Check sheet for the modelled part. Datum: model origin and axes. Units: mm. A direction names the side the tool comes from. Round coordinates to 2 decimals unless told otherwise and drop trailing zeros. Order: outer loops, then holes, each group sorted by start corner. A loop starts at its lowest first (then second) coordinate and runs counter-clockwise, first axis right, second up.
from build123d import *

# Parameters (mm, degrees)
SKETCH028_W     = 110
SKETCH028_H     = 32.6
PAD019_DEPTH    = 46
POCKET009_DEPTH = 19.35
SKETCH030_R     = 2.25
POCKET010_DEPTH = 5
FILLET008_R     = 3.5
SKETCH031_W     = 97
SKETCH031_H     = 2.5
POCKET011_DEPTH = 14.4
FILLET009_R     = 2
FILLET010_R     = 5
SKETCH032_W     = 25.7
SKETCH032_H     = 12.8
POCKET012_DEPTH = 11.6
SKETCH033_W     = 6.52
SKETCH033_H     = 12.8
SKETCH033_W_2   = 6.6
POCKET013_DEPTH = 22
SKETCH034_W     = 6.6
SKETCH034_H     = 15.25
SKETCH034_W_2   = 6.52
POCKET014_DEPTH = 17.55
FILLET011_R     = 1.5
SKETCH035_R     = 1.6
POCKET015_DEPTH = 5
SKETCH036_W     = 5.6
SKETCH036_H     = 2.6
POCKET016_DEPTH = 8.3
SKETCH037_W     = 5.6
SKETCH037_H     = 2.6
POCKET017_DEPTH = 8.3
PRISM_DEPTH     = 56


with BuildPart() as part:
    # Sketch028 → Pad019 (new body)
    with BuildSketch(Plane.XY):
        Rectangle(SKETCH028_W, SKETCH028_H)
    extrude(amount=PAD019_DEPTH)

    # Sketch029 (on Face6 of Pad019) → Pocket009 (cut)
    with BuildSketch(Plane.XY.offset(46)):
        Polygon((-50.7, 16.3), (-42, 16.3), (-42, 11.3), (-33, 11.3), (-33, 16.3), (33, 16.3), (33, 11.3), (42, 11.3), (42, 16.3), (50.7, 16.3), (50.7, -13.8), (-50.7, -13.8), align=None)
    extrude(amount=-POCKET009_DEPTH, mode=Mode.SUBTRACT)

    # Sketch030 (on Face1 of Pocket009) → Pocket010 (cut)
    with BuildSketch(Plane(origin=(0, 16.3, 0), x_dir=(-1, 0, 0), z_dir=(0, 1, 0))):
        with Locations((-37.5, 41.5)):
            Circle(SKETCH030_R)
        with Locations((37.5, 41.5)):
            Circle(SKETCH030_R)
    extrude(amount=-POCKET010_DEPTH, mode=Mode.SUBTRACT)

    # Fillet008
    fillet008_edges = [part.edges().sort_by_distance(p)[0] for p in [
        (33, 13.8, 46),
        (-33, 13.8, 46),
        (-42, 13.8, 46),
        (42, 13.8, 46),
    ]]
    fillet(fillet008_edges, radius=FILLET008_R)

    # Sketch031 (on Face8 of Fillet008) → Pocket011 (cut)
    with BuildSketch(Plane.XY.offset(46)):
        with Locations((0, -15.05)):
            Rectangle(SKETCH031_W, SKETCH031_H)
    extrude(amount=-POCKET011_DEPTH, mode=Mode.SUBTRACT)

    # Fillet009
    fillet009_edges = [part.edges().sort_by_distance(p)[0] for p in [
        (48.5, -15.05, 31.6),
        (-48.5, -15.05, 31.6),
    ]]
    fillet(fillet009_edges, radius=FILLET009_R)

    # Fillet010
    fillet010_edges = [part.edges().sort_by_distance(p)[0] for p in [
        (42, 13.8, 26.65),
        (-33, 13.8, 26.65),
        (33, 13.8, 26.65),
        (-42, 13.8, 26.65),
    ]]
    fillet(fillet010_edges, radius=FILLET010_R)

    # Sketch032 (on Face1 of Fillet010) → Pocket012 (cut)
    with BuildSketch(Plane.XY.offset(26.65)):
        with Locations((13.55, -5)):
            Rectangle(SKETCH032_W, SKETCH032_H)
    extrude(amount=-POCKET012_DEPTH, mode=Mode.SUBTRACT)

    # Sketch033 (on Face38 of Pocket012) → Pocket013 (cut)
    with BuildSketch(Plane.XY.offset(15.05)):
        with Locations((5.51, -5)):
            Rectangle(SKETCH033_W, SKETCH033_H)
        with Locations((21.58, -5)):
            Rectangle(SKETCH033_W_2, SKETCH033_H)
    extrude(amount=-POCKET013_DEPTH, mode=Mode.SUBTRACT)

    # Sketch034 (on Face2 of Pocket013) → Pocket014 (cut)
    with BuildSketch(Plane(origin=(0, 16.3, 0), x_dir=(-1, 0, 0), z_dir=(0, 1, 0))):
        with Locations((-21.58, 7.625)):
            Rectangle(SKETCH034_W, SKETCH034_H)
        with Locations((-5.51, 7.625)):
            Rectangle(SKETCH034_W_2, SKETCH034_H)
    extrude(amount=-POCKET014_DEPTH, mode=Mode.SUBTRACT)

    # Fillet011
    fillet011_edges = [part.edges().sort_by_distance(p)[0] for p in [
        (0.7, 1.4, 20.85),
        (26.4, -11.4, 20.85),
        (0.7, -11.4, 20.85),
        (26.4, 1.4, 20.85),
        (24.88, 16.3, 7.625),
        (18.28, 16.3, 7.625),
        (8.77, 16.3, 7.625),
        (2.25, 16.3, 7.625),
    ]]
    fillet(fillet011_edges, radius=FILLET011_R)

    # Sketch035 (on Face31 of Fillet011) → Pocket015 (cut)
    with BuildSketch(Plane(origin=(0, 0, 0), x_dir=(1, 0, 0), z_dir=(0, 0, -1))):
        with Locations((-37.5, 11.5)):
            Circle(SKETCH035_R)
        with Locations((-37.5, -11.5)):
            Circle(SKETCH035_R)
        with Locations((37.5, -11.5)):
            Circle(SKETCH035_R)
        with Locations((37.5, 11.5)):
            Circle(SKETCH035_R)
    extrude(amount=-POCKET015_DEPTH, mode=Mode.SUBTRACT)

    # Sketch036 (on Face10 of Pocket015) → Pocket016 (cut)
    with BuildSketch(Plane(origin=(0, 16.3, 0), x_dir=(-1, 0, 0), z_dir=(0, 1, 0))):
        with Locations((-37.5, 3.8)):
            Rectangle(SKETCH036_W, SKETCH036_H)
        with Locations((37.5, 3.8)):
            Rectangle(SKETCH036_W, SKETCH036_H)
    extrude(amount=-POCKET016_DEPTH, mode=Mode.SUBTRACT)

    # Sketch037 (on Face65 of Pocket015) → Pocket017 (cut)
    with BuildSketch(Plane.XZ.offset(16.3)):
        with Locations((-37.5, 3.8)):
            Rectangle(SKETCH037_W, SKETCH037_H)
        with Locations((37.5, 3.8)):
            Rectangle(SKETCH037_W, SKETCH037_H)
    extrude(amount=-POCKET017_DEPTH, mode=Mode.SUBTRACT)

    # Prism → Prism (cut)
    with BuildSketch(Plane(origin=(-28, 16.3, 26.65), x_dir=(0, 0.707107, 0.707107), z_dir=(1, 0, 0))):
        Polygon((16, 0), (-8, 13.856406), (-8, -13.856406), align=None)
    extrude(amount=PRISM_DEPTH, mode=Mode.SUBTRACT)


solid = part.part
1) Sectioned sample at C-C on x = -37.5. Record the cut outline in (y, z).
2) Gauge pin test, flat ends, axial feed: pin 1 (10.5 mm diameter, centred on x = 7.5, y = 6, fed in from -Z); pin 2 (3 mm diameter, centred on x = 30, y = -7.5, fed in from +Z); pin 3 (0.8 mm diameter, centred on x = 1.5, y = -7.5, fed in from +Z); pin 4 (5 mm diameter, centred on x = 21, z = 35.5, fed in from -Y). Record the tip position at first contact, or that the pin passes through.
3) Sectioned sample at D-D on y = -7. Record the cut outline in (x, z).
4) Scan lines: line 1 (X direction, y = 11.5, z = 1.8); line 2 (X direction, y = 0, z = 5); line 3 (Y direction, x = -37.5, z = 1.3). Record each from-to range of solid material in increasing order.
5) Set-up check for faces 1 (the face through (6, 9, 15.25)), 2 (the face through (-38.16, -13.13, 2.5)), 3 (the face through (34.05, 13.76, 45)), 4 (the face through (-40.3, 12, 4)): record each of +Z, -Z, +X, -X, +Y, -Y from which the full face is reachable in a straight line by a thin tool's end or side.
6) Sectioned sample at A-A on x = 7.5. Record the cut outline in (y, z), and give its area (3 significant figures).
7) Sectioned sample at B-B on z = 41.5. Record the cut outline in (x, y), and give its area (3 significant figures).
8) Draft check along X on faces 5 (the face through (-53, 0, 46)), 6 (the face through (36.84, -13.13, 2.5)), 7 (the face through (55, 0, 23)). Enter one of: pulls with the +X half, pulls with the -X half, needs draft (parallel to the pull), parting line crosses it, or undercut.
Values found:
1. outline: (-16.3, 0) - (-13.1, 0) - (-13.1, 2.5) - (-16.3, 2.5) - close; (-16.3, 5.1) - (-8, 5.1) - (-8, 2.5) - (-9.9, 2.5) - (-9.9, 0) - (9.9, 0) - (9.9, 2.5) - (8, 2.5) - (8, 5.1) - (16.3, 5.1) - (16.3, 39.25) - (11.3, 39.25) - (11.3, 26.65) - (-13.8, 26.65) - (-13.8, 31.6) - (-16.3, 31.6) - close; (11.3, 43.75) - (16.3, 43.75) - (16.3, 46) - (11.3, 46) - close; (13.1, 0) - (16.3, 0) - (16.3, 2.5) - (13.1, 2.5) - close
2. pin 1: stops at z = 0
2. pin 2: stops at z = 26.65
2. pin 3: stops at z = 15.05
2. pin 4: passes through
3. outline: (-55, 0) - (2.25, 0) - (2.25, 15.05) - (0.7, 15.05) - (0.7, 26.65) - (-50.7, 26.65) - (-50.7, 46) - (-55, 46) - close; (8.77, 0) - (18.28, 0) - (18.28, 15.05) - (8.77, 15.05) - close; (24.88, 0) - (55, 0) - (55, 46) - (50.7, 46) - (50.7, 26.65) - (26.4, 26.65) - (26.4, 15.05) - (24.88, 15.05) - close
4. line 1: x = -55 to -39.1, -35.9 to 2.25, 8.77 to 18.28, 24.88 to 35.9, 39.1 to 55
4. line 2: x = -55 to 2.25, 8.77 to 18.28, 24.88 to 55
4. line 3: y = -16.3 to -13.1, -9.9 to 9.9, 13.1 to 16.3
5. face 1: -Z, +Y
5. face 2: -Y
5. face 3: +Z, +Y, -Y
5. face 4: +Y
6. outline: (-16.3, 0) - (-11.4, 0) - (-11.4, 26.65) - (-13.8, 26.65) - (-13.8, 31.6) - (-16.3, 31.6) - close; (1.4, 15.25) - (16.3, 15.25) - (16.3, 15.34) - (4.99, 26.65) - (1.4, 26.65) - close
6. area: 249 mm2
7. outline: (-55, -16.3) - (-48.5, -16.3) - (-48.5, -13.8) - (-50.7, -13.8) - (-50.7, 16.3) - (-55, 16.3) - close; (-42, 11.3) - (-39.75, 11.3) - (-39.75, 16.3) - (-42, 16.3) - close; (-35.25, 11.3) - (-33, 11.3) - (-33, 16.3) - (-35.25, 16.3) - close; (33, 11.3) - (35.25, 11.3) - (35.25, 16.3) - (33, 16.3) - close; (39.75, 11.3) - (42, 11.3) - (42, 16.3) - (39.75, 16.3) - close; (48.5, -16.3) - (55, -16.3) - (55, 16.3) - (50.7, 16.3) - (50.7, -13.8) - (48.5, -13.8) - close
7. area: 336 mm2
8. face 5: needs draft
8. face 6: undercut
8. face 7: pulls with the +X half
